For this review, use the dimensioned drawing (mm, ordinates from the lowest corner) and the shaded views. A direction names the side the tool comes from. Coordinates: 2 decimals unless noted, no trailing zeros. Write each loop counter-clockwise with the first axis right and the second up, starting at its lowest first coordinate (ties: lowest second). Pieces come first, ordered by that corner, then holes. Notation, with made-up numbers: (17, -3) - (52, -3) arc R19 cw to (52, 2) - close; hole circle Ø6 at (24, 51). An arc over 180 degrees is marked (long way). Answer as a JSON object with one key per item and string values.
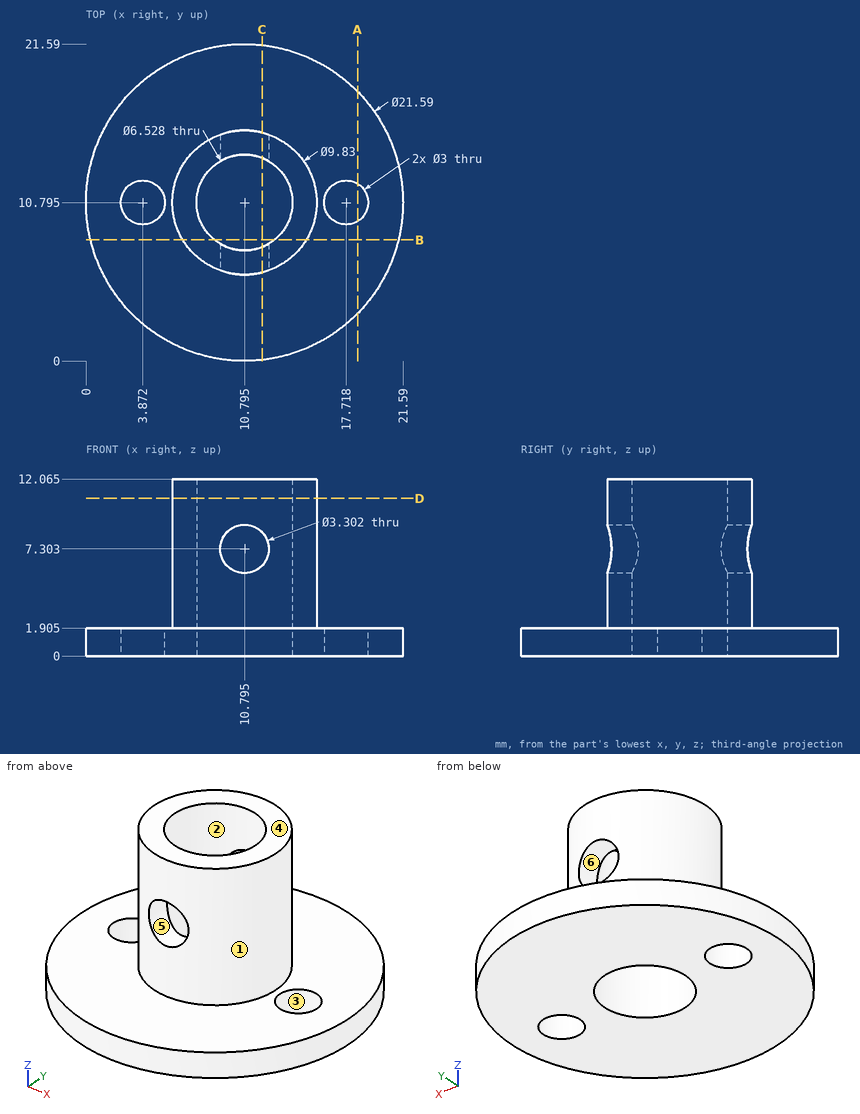
(1) For pin 1 (5 mm diameter, centred on y = 12.5, z = 4.5, fed in from +X); pin 2 (4 mm diameter, centred on x = 10.8, z = 7.3, fed in from +Y); pin 3 (6 mm diameter, centred on y = 12, z = 9.5, fed in from -X); pin 4 (2 mm diameter, centred on x = 10.8, z = 7.3, fed in from -Y), all flat-tipped, find the tip position at first contact; note any pin that passes through.
Solved:
{"pin 1": "stops at x = 15.71", "pin 2": "stops at y = 15.71", "pin 3": "stops at x = 5.88", "pin 4": "passes through"}
(2) To check wall thickness, follow line 1 (Y direction, x = 13, z = 0.75) (1 decimal); line 2 (Y direction, x = 5, z = 0.5) (1 decimal); line 3 (Z direction, x = 4.5, y = 13.5) (1 decimal). State the ranges of each line that lie inside material, in increasing order. Write a range as from..to.
Solved:
{"line 1": "y = 0.2..8.4, 13.2..21.4", "line 2": "y = 1.7..9.8, 11.8..19.9", "line 3": "z = 0..1.9"}
(3) Take a section at D-D, the plane z = 10.75. Write out the cut boundary in (x, y) (1 decimal).
Solved:
{"outline": "circle Ø9.8 at (10.8, 10.8); hole circle Ø6.5 at (10.8, 10.8)"}
(4) Tool access review of the marked faces 1 and 2: name each direction out of +Z, -Z, +X, -X, +Y, -Y from which nothing blocks a thin tool from reaching the whole face with its end or side.
Solved:
{"face 1": "+Z", "face 2": "+Z, -Z"}
(5) Take a section at A-A, the plane x = 18.5. Write out the cut boundary in (y, z) (1 decimal).
Solved:
{"outline": "(3.2, 0) - (9.5, 0) - (9.5, 1.9) - (3.2, 1.9) - close; (12.1, 0) - (18.4, 0) - (18.4, 1.9) - (12.1, 1.9) - close"}
(6) Take a section at B-B, the plane y = 8.25. Write out the cut boundary in (x, z) (1 decimal).
Solved:
{"outline": "(0.3, 0) - (8.8, 0) - (8.8, 12.1) - (6.6, 12.1) - (6.6, 1.9) - (0.3, 1.9) - close; (12.8, 0) - (21.3, 0) - (21.3, 1.9) - (15, 1.9) - (15, 12.1) - (12.8, 12.1) - close"}
(7) Take a section at C-C, the plane x = 12. Write out the cut boundary in (y, z) (1 decimal).
Solved:
{"outline": "(0.1, 0) - (7.8, 0) - (7.8, 6.2) - (6, 6.2) - (6, 1.9) - (0.1, 1.9) - close; (6, 8.4) - (7.8, 8.4) - (7.8, 12.1) - (6, 12.1) - close; (13.8, 0) - (21.5, 0) - (21.5, 1.9) - (15.6, 1.9) - (15.6, 6.2) - (13.8, 6.2) - close; (13.8, 8.4) - (15.6, 8.4) - (15.6, 12.1) - (13.8, 12.1) - close"}
(8) The part is to be moulded in two halves that separate along Z. For the marked faces 3, 4, 5 and 6, say which applies: pulls with the +Z half, pulls with the -Z half, needs draft (parallel to the pull), parting line crosses it, or undercut.
Solved:
{"face 3": "needs draft", "face 4": "pulls with the +Z half", "face 5": "undercut", "face 6": "undercut"}
